Could you check a few things on this model? Use its own coordinates, in mm. Give positions to 0.01 mm unless a question says otherwise; leave off trailing zeros. Write each loop counter-clockwise with the first axis right and the second up, starting at its lowest first coordinate (ties: lowest second). Pieces come first, ordered by that corner, then holes. Notation, with made-up numbers: M -36.75,22 L 12.25,22 A20 cw 12.25,59 Z; hole C -12,9.5 d11. An arc over 180 degrees is marked long. One line per item, written item: value.
```python
from build123d import *

# Parameters (mm, degrees)
SKETCH_1_R      = 6
EXTRUDE_1_DEPTH = 800
SKETCH_2_R      = 6
EXTRUDE_2_DEPTH = 270
REVOLVE_1_ANGLE = 180
REVOLVE_2_ANGLE = 180


with BuildPart() as part:
    # Sketch 1 → Extrude 1 (new body)
    with BuildSketch(Plane(origin=(0, 0, 0), x_dir=(1, 0, 0), z_dir=(0, 1, 0))):
        with Locations(Location((0, 0, 0), (0, 0, 270))):
            Circle(SKETCH_1_R)
    extrude(amount=EXTRUDE_1_DEPTH)

    # Sketch 2 → Extrude 2 (add, symmetric)
    with BuildSketch(Plane(origin=(0, 0, 0), x_dir=(0, 0, -1), z_dir=(1, 0, 0))):
        with Locations((0, 600)):
            Circle(SKETCH_2_R)
    extrude(amount=EXTRUDE_2_DEPTH, both=True)

    # Sketch 3 → Revolve 1 (revolve)
    with BuildSketch(Plane(origin=(270, 0, 0), x_dir=(0, 0, -1), z_dir=(1, 0, 0))):
        with BuildLine():
            Line((0, 606), (0, 594))
            ThreePointArc((0, 594), (6, 600), (0, 606))
        make_face()
    revolve_1 = revolve(axis=Axis((270, 606, 0), (0, -1, 0)), revolution_arc=REVOLVE_1_ANGLE)

    # Sketch 4 → Revolve 2 (revolve)
    with BuildSketch(Plane(origin=(0, 800, 0), x_dir=(1, 0, 0), z_dir=(0, 1, 0))):
        with BuildLine():
            Line((0, 6), (0, -6))
            ThreePointArc((0, -6), (6, 0), (0, 6))
        make_face()
    revolve(axis=Axis((0, 800, -6), (0, 0, 1)), revolution_arc=REVOLVE_2_ANGLE)

    # Mirror 1: Revolve 1 across plane
    add(revolve_1.mirror(Plane(origin=(0, 0, 0), x_dir=(0, 0, 1), z_dir=(1, 0, 0))))


solid = part.part
```
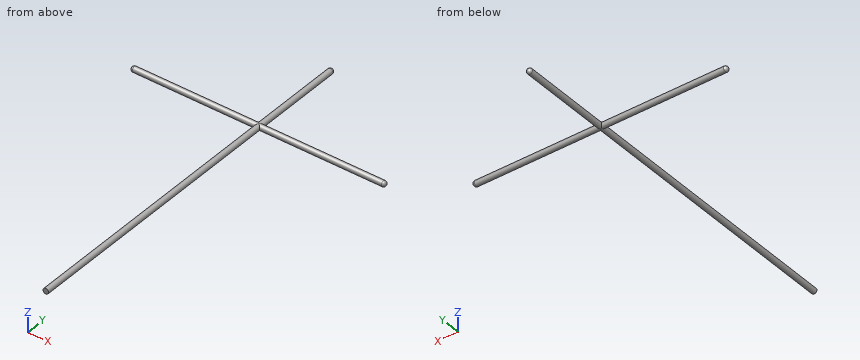
1) I'm going to push flat-ended pins straight in: pin 1 (1.5 mm diameter, centred on x = -188.5, z = 3.5, fed in from +Y); pin 2 (1 mm diameter, centred on x = -103.5, z = -4, fed in from -Y); pin 3 (3 mm diameter, centred on y = 470.5, z = -2.5, fed in from -X). Where does each tip first touch, or does it pass through?
Outcome:
pin 1: stops at y = 605.33
pin 2: stops at y = 595.13
pin 3: stops at x = -5.92
2) If we section it at A-A, the plane z = 0: Write out the boundary of the cut face in (x, y), then the cut area to 3 significant figures.
Outcome:
outline: M -270,594 L -6,594 L -6,0 L 6,0 L 6,594 L 270,594 A6 ccw 270,606 L 6,606 L 6,800 A6 ccw -6,800 L -6,606 L -270,606 A6 ccw Z
area: 16,100 mm^2
3) If we section it at B-B, the plane x = 212: Write out the boundary of the cut face in (y, z).
Outcome:
outline: C 600,0 d12
4) Please list where these lines run through material, in increasing order: L1, parallel to Y at x = -101.5, z = -0.5; L2, parallel to X at y = 341, z = -1.5; L3, parallel to X at y = 394.5, z = -0.25. Write a range as from..to.
Outcome:
L1: y = 594.02..605.98
L2: x = -5.81..5.81
L3: x = -5.99..5.99
5) If we section it at C-C, the plane y = 377: Write out the boundary of the cut face in (x, z).
Outcome:
outline: C 0,0 d12
